Geometry: final body of the model. Coordinates: model frame, mm. A direction names the side the tool comes from. Round coordinates to 2 decimals unless told otherwise and drop trailing zeros. Write each loop counter-clockwise with the first axis right and the second up, starting at its lowest first coordinate (ties: lowest second). Pieces come first, ordered by that corner, then holes. Notation, with made-up numbers: (7, 40) -> (30, 40) arc R23 cw to (30, 54) -> close; hole circle Ø8 at (60, 42.25). An arc over 180 degrees is marked (long way). Use one line per item in the form item = value. Start each with the question number.
1. Pin query (flat end, axial travel): pin 1 Ø5 at (y, z) = (-9.81, -10.21) entering from -X; pin 2 Ø1.5 at (x, y) = (1, -34.5) entering from -Z; pin 3 Ø4 at (x, z) = (-2.5, -9) entering from +Y. Return the tip coordinate at first contact, or that it passes through.
2. Reachability of faces 1 (the face through (3.86, -59.17, -0.85)), 2 (the face through (-1, -40, -20)), 3 (the face through (2, -11, -40)) from +Z, -Z, +X, -X, +Y, -Y: full face, straight path, thin tool, end or side. Return the list, or none.
3. Cut plane C-C, the plane y = -56. Return the cut outline in (x, z).
4. Line query: L1, parallel to Y at x = 3.4, z = -30; L2, parallel to X at y = -45, z = -42; L3, parallel to Y at x = -2.55, z = -30. Output: solid intervals per line, ascending.
5. Cut plane B-B, the plane y = -30. Return the cut outline in (x, z), plus the area to 3 significant figures.
6. Draft query along Y for faces 4 (the face through (0.25, -30.31, -49.96)), 5 (the face through (1.875, -48.646, -8.443)), 6 (the face through (3.86, -59.15, -59.17)), 7 (the face through (2.89, -48.14, -50.97)). Return one class per face: pulls with the +Y half, pulls with the -Y half, needs draft (parallel to the pull), parting line crosses it, or undercut.
7. Cut plane D-D, the plane y = -50. State how many separate pieces and enclosed holes the cut face has, plus the area to 3 significant figures.
Autodesk Fusion 360 part; units mm, degrees
sketch "Sketch1" plane through (0, 0, 0) normal (1, 0, 0) x (0, 0, -1)
  line L0 (0, 0) -> (0, -60)
  line L1 (0, -60) -> (60, -60)
  line L2 (60, -60) -> (60, -40)
  line L3 (40, 0) -> (0, 0)
  line L4 (40, -40) -> (40, -60)
  line L5 (40, -40) -> (0, -40)
  line L6 (60, -40) -> (40, -20)
  line L7 (40, -20) -> (40, 0)
  line L8 (60, -50) -> (0, -50) construction
  line L9 (10.2088, 0) -> (10.2088, -60) construction
  line L10 (0, -9.7462) -> (40, -10) construction
  line L11 (0, -30) -> (50, -30) construction
  line L12 (49.9986, -60) -> (50, -30) construction
  line L13 (30, -60) -> (30, 0) construction
  circle A0 centre (10.2088, -9.811) radius 2.1
  circle A1 centre (10.2088, -30) radius 2.1
  circle A2 centre (10.2088, -50) radius 2.1
  circle A3 centre (30, -50) radius 2.1
  circle A4 centre (49.9991, -50) radius 2.1
  circle A5 centre (30, -50) radius 4.1
  circle A6 centre (10.2088, -50) radius 4.1
  dimension "d1" = 60
  dimension "d2" = 60
  dimension "d3" = 20
  dimension "d4" = 20
  dimension "d15" = 4.2
  dimension "d16" = 4.2
  dimension "d17" = 4.2
  dimension "d18" = 4.2
  dimension "d19" = 4.2
  dimension "d20" = 8.2
  dimension "d21" = 8.2
extrude "Extrude1" add sketch "Sketch1" along normal blind 4 contours L0 L1 L2 L3 L4 L5 L6 L7 | L0 L1 L4 L5 | A5 | A6
extrude "Extrude2" add sketch "Sketch1" against normal blind 5 contours L0 L1 L4 L5
chamfer "Chamfer1" distance 2 angle 45 5 edges at (0, -9.0516, -8.2509) (0, -29.2406, -8.2509) (0, -49.2406, -8.2509) (0, -49.2406, -28.0421) (0, -49.2406, -48.0412)
fillet "Fillet1" radius 2 9 edges at (2, -60, -60) (-0.5, -60, 0) (2, -40, -60) (2, -20, -40) (2, 0, -40) (2, 0, 0) (-2.5, -40, -40) (-2.5, -60, -40) (-2.5, -40, 0)
chamfer "Chamfer2" distance 0.5 angle 45 25 edges at (-5, -51.4826, -26.1775) (-5, -51.4826, -6.3862) (0, -60, -48) (0, -59.4142, -59.4142) (0, -49.4142, -60) (0, -40.0631, -59.8478) (0, -30, -50) (0, -19.9369, -40.1522) (0, -10.5858, -40) (0, -0.5858, -39.4142) (0, 0, -20) (0, -0.5858, -0.5858) (0, -22, 0) (4, -59.4142, -59.4142) (4, -49.4142, -60) (4, -40.0631, -59.8478) (4, -30, -50) (4, -19.9369, -40.1522) (4, -10.5858, -40) (4, -0.5858, -39.4142) (4, 0, -20) (4, -0.5858, -0.5858) (4, -30, 0) (4, -59.4142, -0.5858) (4, -60, -30)
chamfer "Chamfer3" distance 0.2 angle 45 5 edges at (4, -9.0516, -8.2509) (4, -29.2406, -8.2509) (4, -49.2406, -8.2509) (4, -49.2406, -28.0421) (4, -49.2406, -48.0412)
chamfer "Chamfer4" distance 2 angle 45 8 edges at (-5, -59.4142, -0.5858) (-5, -50, 0) (-5, -40.5858, -0.5858) (-5, -40, -20) (-5, -40.5858, -39.4142) (-5, -50, -40) (-5, -59.4142, -39.4142) (-5, -60, -20)
Outcome:
q1.pin_1 = 1.6
q1.pin_2 = -55.25
q1.pin_3 = -40
q2.face_1 = +Z, +X, -Y
q2.face_2 = +Z, -Z, -X, +Y
q2.face_3 = -Z, +X, -X, +Y
q3.outline = (-5, -38) -> (-3, -40) -> (0, -40) -> (0, -59.5) -> (0.5, -60) -> (3.5, -60) -> (4, -59.5) -> (4, -0.5) -> (3.5, 0) -> (-3, 0) -> (-5, -2) -> close
q4.L1 = -60 to -52.1, -47.9 to 0
q4.L2 = 0 to 4
q4.L3 = -60 to -54.1, -45.9 to -40
q5.outline = (0, -49.29) -> (0.5, -50) -> (3.5, -50) -> (4, -49.29) -> (4, -12.51) -> (3.8, -12.31) -> (2, -12.31) -> (0, -14.31) -> close; (0, -6.11) -> (2, -8.11) -> (3.8, -8.11) -> (4, -7.91) -> (4, -0.5) -> (3.5, 0) -> (0.5, 0) -> (0, -0.5) -> close
q5.area = 179 mm^2
q6.face_4 = pulls with the +Y half
q6.face_5 = undercut
q6.face_6 = pulls with the -Y half
q6.face_7 = undercut
q7.separate_pieces = 4
q7.enclosed_holes = 0
q7.area = 291 mm^2
